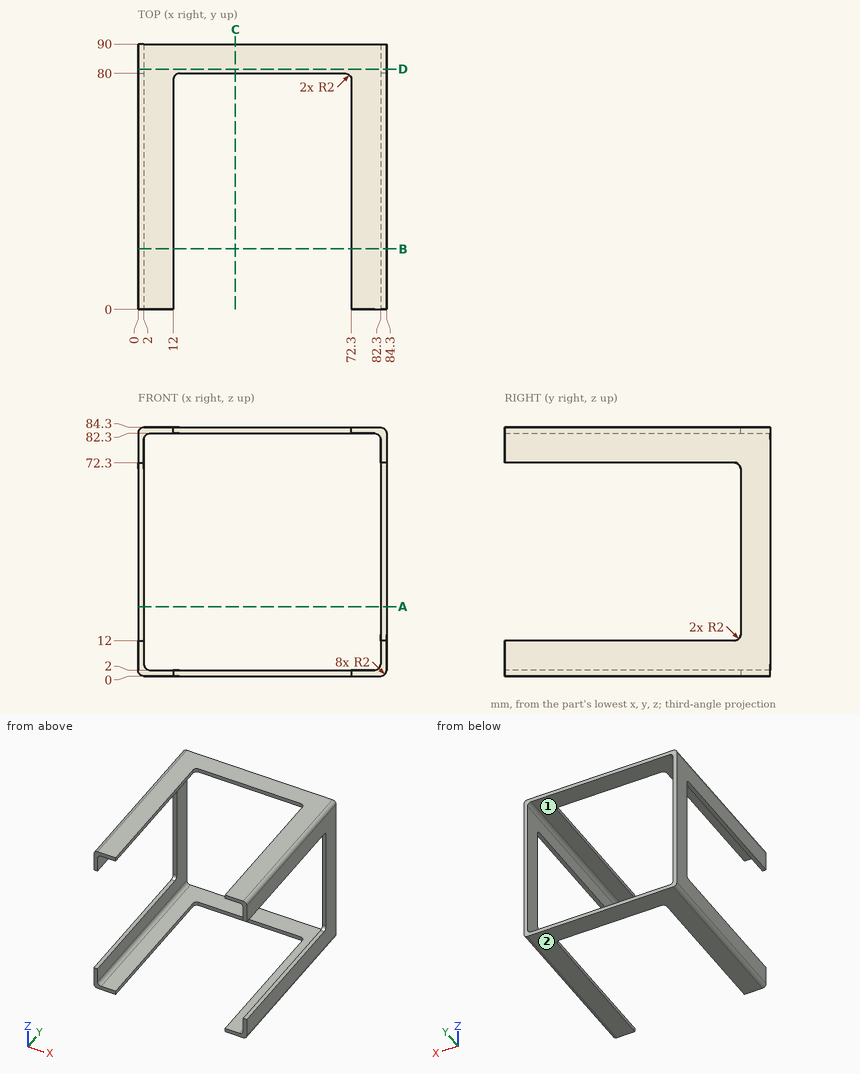
Source: three-view drawing plus pictorial views. Frame: mm from the lowest corner of the part. Round coordinates to 2 decimals unless told otherwise and drop trailing zeros. Loops run counter-clockwise (first coordinate to the right, second up) from the corner with the lowest first, then second, coordinate; pieces in that order, holes last.
Q1. Section C-C, the plane x = 33. Return loops of the section in (y, z), plus the area to 3 significant figures.
Q2. Ray query, line 1 (X direction, y = 82.5, z = 32). Return the intervals inside material, ascending.
Q3. Section A-A, the plane z = 23.5. Return loops of the section in (x, y).
Q4. First-contact query: P1, Ø2, axis at x = 0.5, y = 57, coming from the -Z side; P2, Ø1, axis at x = 84, y = 29, coming from the -Z side; P3, Ø2, axis at y = 51.5, z = 0.5, coming from the -X side. Flat tips, straight axial feed; report the tip coordinate or a pass-through.
Q5. Section D-D, the plane y = 81.5. Return loops of the section in (x, z).
Q6. Section B-B, the plane y = 20.5. State how many separate pieces and enclosed holes the cut face has, plus the area to 3 significant figures.
Q7. Mould query, pull axis X, two halves, no side actions, for the marked faces 1 and 2. Classes: pulls with the +X half, pulls with the -X half, needs draft (parallel to the pull), parting line crosses it, or undercut.
Solutions:
1. outline: (80, 0) - (90, 0) - (90, 2) - (80, 2) - close; (80, 82.3) - (90, 82.3) - (90, 84.3) - (80, 84.3) - close
1. area: 40.0 mm2
2. line 1: x = 0 to 2, 82.3 to 84.3
3. outline: (0, 80) - (2, 80) - (2, 90) - (0, 90) - close; (82.3, 80) - (84.3, 80) - (84.3, 90) - (82.3, 90) - close
4. P1: stops at z = 0.06
4. P2: stops at z = 0.4
4. P3: stops at x = 0.06
5. outline: (0, 2) arc R2 ccw to (2, 0) - (82.3, 0) arc R2 ccw to (84.3, 2) - (84.3, 82.3) arc R2 ccw to (82.3, 84.3) - (2, 84.3) arc R2 ccw to (0, 82.3) - close; hole (2, 4) arc R2 ccw to (4, 2) - (80.3, 2) arc R2 ccw to (82.3, 4) - (82.3, 80.3) arc R2 ccw to (80.3, 82.3) - (4, 82.3) arc R2 ccw to (2, 80.3) - close
6. separate pieces: 4
6. enclosed holes: 0
6. area: 176 mm2
7. face 1: undercut
7. face 2: needs draft
